```python
from build123d import *

# Parameters (mm, degrees)
BOSS_EXTRUDE1_DEPTH = 85
SKETCH3_R           = 11.5
SKETCH3_R_2         = 4.5
SKETCH3_R_3         = 2.15
CUT_EXTRUDE1_DEPTH  = 85
SKETCH4_R           = 1.6
CUT_EXTRUDE2_DEPTH  = 85


with BuildPart() as part:
    # Sketch2 → Boss-Extrude1 (new body)
    with BuildSketch(Plane.XY):
        Polygon((0, 0), (0, 86.2), (-10, 86.2), (-10, -4.142135624), align=None)
    extrude(amount=BOSS_EXTRUDE1_DEPTH)

    # Sketch3 → Cut-Extrude1 (cut)
    with BuildSketch(Plane.ZY.offset(10)):
        with Locations(Location((42.5, 46.2, 0), (0, 0, 270))):
            Circle(SKETCH3_R)
        with Locations(Location((42.5, 65.45, 0), (0, 0, 270))):
            Circle(SKETCH3_R_2)
        with Locations(Location((42.5, 75.2, 0), (0, 0, 270))):
            Circle(SKETCH3_R_3)
        with Locations(Location((67.61473671, 31.7, 0), (0, 0, 270))):
            Circle(SKETCH3_R_3)
        with Locations(Location((17.38526329, 31.7, 0), (0, 0, 270))):
            Circle(SKETCH3_R_3)
    extrude(amount=-CUT_EXTRUDE1_DEPTH, mode=Mode.SUBTRACT)

    # Sketch4 → Cut-Extrude2 (cut)
    with BuildSketch(Plane(origin=(0, 0, 0), x_dir=(0, 0, -1), z_dir=(1, 0, 0))):
        with Locations((-65, 8.5)):
            Circle(SKETCH4_R)
        with Locations((-20, 8.5)):
            Circle(SKETCH4_R)
        with Locations((-42.5, 8.5)):
            Circle(SKETCH4_R)
    extrude(amount=-CUT_EXTRUDE2_DEPTH, mode=Mode.SUBTRACT)


solid = part.part
```
Can you work these out from the model? Positions are in its coordinate system, mm. Coordinates: 2 decimals unless noted, no trailing zeros. Write each loop counter-clockwise with the first axis right and the second up, starting at its lowest first coordinate (ties: lowest second). Pieces come first, ordered by that corner, then holes. Notation, with made-up numbers: (55, 1) - (101, 1) arc R25 ccw to (101, 21) - close; hole circle Ø10 at (35, 40). An arc over 180 degrees is marked (long way). Return JSON: item names as keys, results as strings.
Q1. If we section it at C-C (x = -2): Count the separate pieces of the cut face and the enclosed holes in it, then the cut area to 3 significant figures.
Computed values:
{"separate pieces": "1", "enclosed holes": "8", "area": "6,850 mm2"}
Q2. Thinking about a two-plate mould opening in Y: for faces 1 (the cylindrical face through (-4.93, 7.89, 63.52)), 2 (the flat face through (-5, 42, 0)), 3 (the flat face through (-5, 86.2, 42)), which applies, +Y half, -Y half, draft (parallel to the pull), parting line (faces both ways), or undercut?
Computed values:
{"face 1": "undercut", "face 2": "draft", "face 3": "+Y half"}
Q3. If we section it at B-B (y = 31.7): Please give me the cut outline in (x, z).
Computed values:
{"outline": "(-10, 0) - (0, 0) - (0, 15.24) - (-10, 15.24) - close; (-10, 19.54) - (0, 19.54) - (0, 65.46) - (-10, 65.46) - close; (-10, 69.76) - (0, 69.76) - (0, 85) - (-10, 85) - close"}
Q4. If we section it at D-D (y = 65.45): Please give me the cut outline in (x, z).
Computed values:
{"outline": "(-10, 0) - (0, 0) - (0, 38) - (-10, 38) - close; (-10, 47) - (0, 47) - (0, 85) - (-10, 85) - close"}
Q5. I'm going to push flat-ended pins straight in: pin 1 Ø3.5 at (y, z) = (8.5, 20) entering from -X; pin 2 Ø1.5 at (x, z) = (-1.5, 33) entering from -Y; pin 3 Ø2.5 at (y, z) = (31.7, 67.61) entering from -X. Where does each tip first touch, or does it pass through?
Computed values:
{"pin 1": "stops at x = -10", "pin 2": "stops at y = -0.93", "pin 3": "passes through"}
Q6. If we section it at A-A (y = 75.2): Please give me the cut outline in (x, z).
Computed values:
{"outline": "(-10, 0) - (0, 0) - (0, 40.35) - (-10, 40.35) - close; (-10, 44.65) - (0, 44.65) - (0, 85) - (-10, 85) - close"}
Q7. Please list where these lines run through material, in increasing order: L1, parallel to Z at x = -5.75, y = 31.7; L2, parallel to Z at x = -5.25, y = 75.2; L3, parallel to Y at x = -2.25, z = 53. Write a range as from..to.
Computed values:
{"L1": "z = 0..15.24, 19.54..65.46, 69.76..85", "L2": "z = 0..40.35, 44.65..85", "L3": "y = -0.93..41.51, 50.89..86.2"}
